Geometry: final body of the model. Coordinates: model frame, mm. Face numbers are marked on the shaded views. A direction names the side the tool comes from. Round coordinates to 2 decimals unless told otherwise and drop trailing zeros. Loops run counter-clockwise (first coordinate to the right, second up) from the corner with the lowest first, then second, coordinate; pieces in that order, holes last. Notation, with made-up numbers: (3.5, 31.25) -> (27.5, 31.25) arc R8 cw to (27.5, 40.25) -> close; hole circle Ø2 at (54.25, -14). An arc over 180 degrees is marked (long way). Answer in a Markdown table with one row per item.
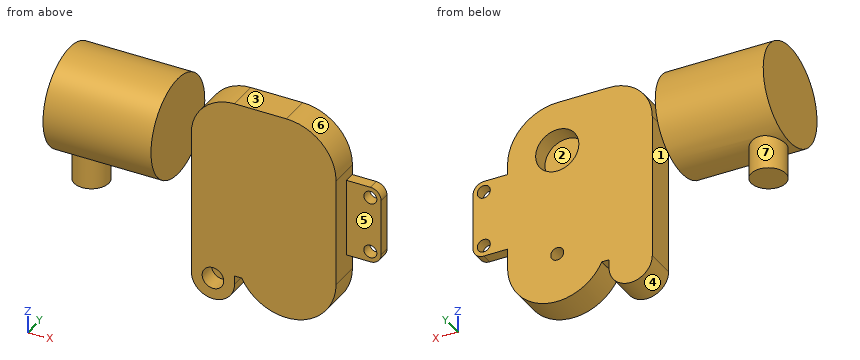
```python
from build123d import *

# Parameters (mm, degrees)
BOSS_EXTRUDE1_DEPTH = 7
SKETCH2_R           = 2.5
CUT_EXTRUDE1_DEPTH  = 4
SKETCH3_R           = 1.5
SKETCH3_R_2         = 5
CUT_EXTRUDE2_DEPTH  = 4
SKETCH4_R           = 11.5
BOSS_EXTRUDE2_DEPTH = 25
SKETCH5_R           = 4
BOSS_EXTRUDE3_DEPTH = 11
SKETCH6_R           = 1.5
BOSS_EXTRUDE4_DEPTH = 2.5


with BuildPart() as part:
    # Sketch1 → Boss-Extrude1 (new body)
    with BuildSketch(Plane(origin=(0, 0, 0), x_dir=(1, 0, 0), z_dir=(0, 1, 0))):
        with BuildLine():
            Line((28.5, 13.628059387), (28.5, -11.371940613))
            ThreePointArc((28.5, -11.371940613), (25.131727984, -19.503668597), (17, -22.871940613))
            Line((17, -22.871940613), (5, -22.871940613))
            ThreePointArc((5, -22.871940613), (-2.071067812, -19.943008425), (-5, -12.871940613))
            Line((-5, -12.871940613), (-5, 20.70125692))
            ThreePointArc((-5, 20.70125692), (0, 25.70125692), (5, 20.70125692))
            Line((5, 20.70125692), (5, 18.70125692))
            Line((5, 18.70125692), (6.67950259, 18.70125692))
            ThreePointArc((6.67950259, 18.70125692), (19.604254191, 24.829303072), (28.5, 13.628059387))
        make_face()
    extrude(amount=BOSS_EXTRUDE1_DEPTH)

    # Sketch2 → Cut-Extrude1 (cut)
    with BuildSketch(Plane.XZ):
        with Locations((0, -20.70125692)):
            Circle(SKETCH2_R)
    extrude(amount=-CUT_EXTRUDE1_DEPTH, mode=Mode.SUBTRACT)

    # Sketch3 → Cut-Extrude2 (cut)
    with BuildSketch(Plane(origin=(0, 7, 0), x_dir=(1, 0, 0), z_dir=(0, 1, 0))):
        with Locations((17, 13.628059387)):
            Circle(SKETCH3_R)
        with Locations((17, -11.371940613)):
            Circle(SKETCH3_R_2)
    extrude(amount=-CUT_EXTRUDE2_DEPTH, mode=Mode.SUBTRACT)

    # Sketch4 → Boss-Extrude2 (add)
    with BuildSketch(Plane.ZY.offset(5)):
        with Locations((17.637770726, -5.75)):
            Circle(SKETCH4_R)
    extrude(amount=BOSS_EXTRUDE2_DEPTH)

    # Sketch5 → Boss-Extrude3 (add)
    with BuildSketch(Plane.XY.offset(10)):
        with Locations((-25, -5.75)):
            Circle(SKETCH5_R)
    extrude(amount=-BOSS_EXTRUDE3_DEPTH)

    # Sketch6 → Boss-Extrude4 (add)
    with BuildSketch(Plane(origin=(0, 7, 0), x_dir=(1, 0, 0), z_dir=(0, 1, 0))):
        with BuildLine():
            Line((28.5, 9), (34, 9))
            ThreePointArc((34, 9), (35.767766953, 8.267766953), (36.5, 6.5))
            Line((36.5, 6.5), (36.5, -6.5))
            ThreePointArc((36.5, -6.5), (35.767766953, -8.267766953), (34, -9))
            Line((34, -9), (28.5, -9))
            Line((28.5, -9), (28.5, 9))
        make_face()
        with Locations((34, -6.5)):
            Circle(SKETCH6_R, mode=Mode.SUBTRACT)
        with Locations((34, 6.5)):
            Circle(SKETCH6_R, mode=Mode.SUBTRACT)
    extrude(amount=-BOSS_EXTRUDE4_DEPTH)


solid = part.part
```
Item 1: Section query C-C, the plane x = -25. Output: boundary loops of the cut face in (y, z).
Ans:
| item | result |
|---|---|
| outline | (-9.75, -1) -> (-1.75, -1) -> (-1.75, 6.86) arc R11.5 ccw (long way) to (-9.75, 6.86) -> close |
Item 2: First-contact query: P1, Ø7, axis at y = -8, z = 13.5, coming from the +X side; P2, Ø3, axis at x = -13.5, y = 4.5, coming from the +Z side; P3, Ø9, axis at x = 17, z = 11.37, coming from the +Y side. Flat tips, straight axial feed; report the tip coordinate or a pass-through.
Ans:
| item | result |
|---|---|
| P1 | x = -5 |
| P2 | z = 25.1 |
| P3 | y = 3 |
Item 3: Section query D-D, the plane y = 2. Output: boundary loops of the cut face in (x, z), and give its area (3 significant figures).
Ans:
| item | result |
|---|---|
| outline | (-30, 9.14) -> (-5, 9.14) -> (-5, -20.7) arc R5 ccw to (5, -20.7) -> (5, -18.7) -> (6.68, -18.7) arc R11.5 ccw to (28.5, -13.63) -> (28.5, 11.37) arc R11.5 ccw to (17, 22.87) -> (5, 22.87) arc R10 ccw to (-5, 12.87) -> (-5, 26.13) -> (-30, 26.13) -> close; hole circle Ø5 at (0, -20.7) |
| area | 1,900 mm2 |
Item 4: Set-up query: the marked faces 5, 6 and 7. Return all of +Z, -Z, +X, -X, +Y, -Y with unobstructed straight access to the full face (end or side cutting, diameter ignored); none if empty.
Ans:
| item | result |
|---|---|
| face 5 | +Z, -Z, +X, -Y |
| face 6 | +Z, +X, +Y, -Y |
| face 7 | -Z |
Item 5: Ray query, L1, parallel to Z at x = 17, y = 5.85; L2, parallel to Z at x = 34, y = 5.9; L3, parallel to X at y = 5.8, z = -6.5. Return the intervals inside material, ascending.
Ans:
| item | result |
|---|---|
| L1 | -25.13 to -15.13, -12.13 to 6.37, 16.37 to 22.87 |
| L2 | -9 to -8, -5 to 5, 8 to 9 |
| L3 | -5 to 32.5, 35.5 to 36.5 |
Item 6: Section query A-A, the plane z = 1.5. Output: boundary loops of the cut face in (x, y).
Ans:
| item | result |
|---|---|
| outline | circle Ø8 at (-25, -5.75); (-5, 0) -> (28.5, 0) -> (28.5, 4.5) -> (36.5, 4.5) -> (36.5, 7) -> (-5, 7) -> close |
Item 7: Mould query, pull axis X, two halves, no side actions, for the marked faces 1, 2, 3 and 4. Classes: released by +X, released by -X, zero draft, split by the parting line, or undercut.
Ans:
| item | result |
|---|---|
| face 1 | released by -X |
| face 2 | undercut |
| face 3 | zero draft |
| face 4 | undercut |
Item 8: Section query B-B, the plane y = -5.75. Output: boundary loops of the cut face in (x, z), and give its area (3 significant figures).
Ans:
| item | result |
|---|---|
| outline | (-30, 6.14) -> (-29, 6.14) -> (-29, -1) -> (-21, -1) -> (-21, 6.14) -> (-5, 6.14) -> (-5, 29.14) -> (-30, 29.14) -> close |
| area | 632 mm2 |
